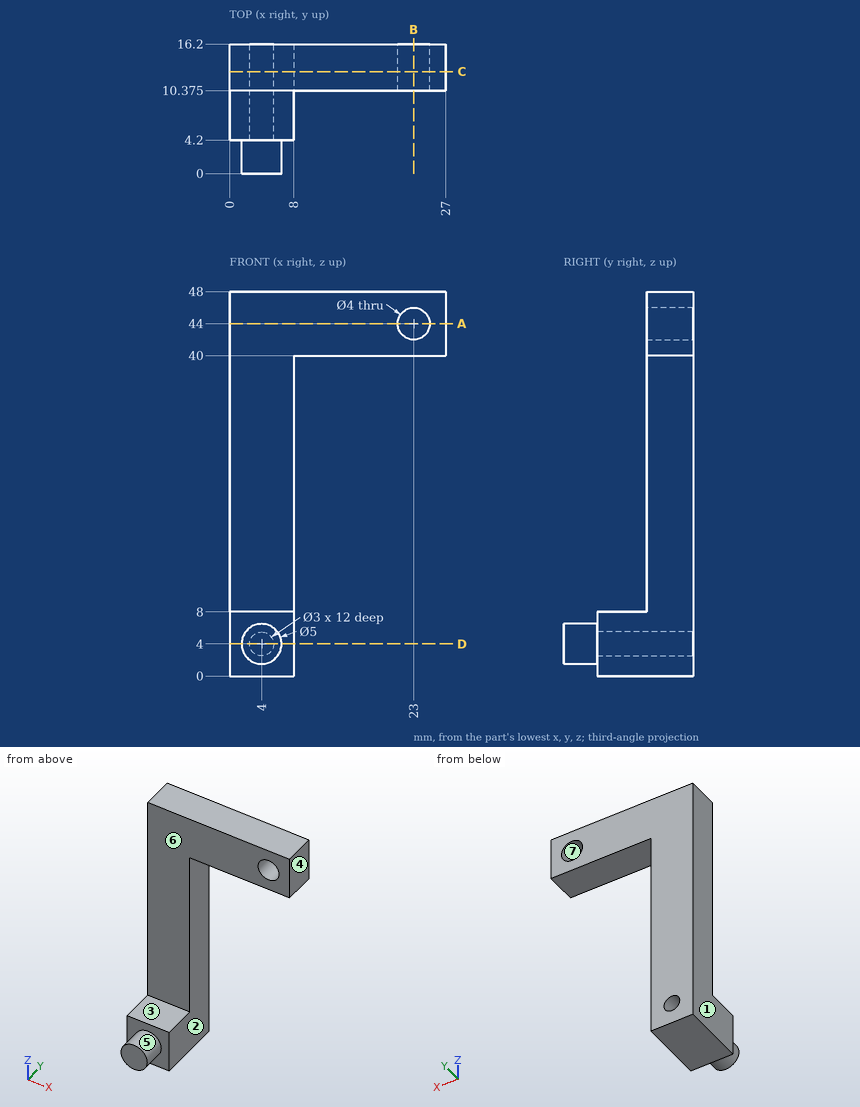
Geometry check sheet. Reference: drawing and pictorial views, mm from the part's lowest x, y, z. A direction names the side the tool comes from. Coordinates: 2 decimals unless noted, no trailing zeros. Order: outer loops, then holes, each group sorted by start corner. A loop starts at its lowest first (then second) coordinate and runs counter-clockwise, first axis right, second up. Notation, with made-up numbers: (-23, -5) -> (0, -5) arc R30 cw to (0, 17) -> close; hole circle Ø2 at (47, 89.25). An arc over 180 degrees is marked (long way). Put each result on its own line as item: value. Start each with the question number.
1) Cross-section at A-A (z = 44). Enter the section's corners in (x, y) (3 decimals), plus the area to 3 significant figures.
2) Cross-section at C-C (y = 12.75). Enter the section's corners in (x, z), plus the area to 3 significant figures.
3) Cross-section at D-D (z = 4). Enter the section's corners in (x, y).
4) Tool access check on the marked faces 1, 2 and 3. Record the directions out of +Z, -Z, +X, -X, +Y, -Y that give a thin tool (end or side, any length) a straight path to the whole face; none if there is none.
5) Material ranges on L1, parallel to X at y = 10.75, z = 4; L2, parallel to X at y = 12.75, z = 44; L3, parallel to Y at x = 16.25, z = 41 (3 decimals), recorded low to high.
6) Go/stop test with flat-tipped pins: pin 1 (3 mm diameter, centred on x = 3.5, y = 7.5, fed in from +Z); pin 2 (3.5 mm diameter, centred on y = 11.5, z = 13.5, fed in from +X); pin 3 (5 mm diameter, centred on x = 9.5, z = 6, fed in from -Y). Record where each tip stops, or that it passes through.
7) Release check for a two-part mould opening along X. For the marked faces 4, 5, 6 and 7 record: pulls with the +X half, pulls with the -X half, needs draft (parallel to the pull), parting line crosses it, or undercut.
8) Cross-section at B-B (x = 23). Enter the section's corners in (y, z) (3 decimals).
Geometry check:
1. outline: (0, 10.375) -> (21, 10.375) -> (21, 16.2) -> (0, 16.2) -> close; (25, 10.375) -> (27, 10.375) -> (27, 16.2) -> (25, 16.2) -> close
1. area: 134 mm^2
2. outline: (0, 0) -> (8, 0) -> (8, 40) -> (27, 40) -> (27, 48) -> (0, 48) -> close; hole circle Ø3 at (4, 4); hole circle Ø4 at (23, 44)
2. area: 516 mm^2
3. outline: (0, 4.2) -> (1.5, 4.2) -> (1.5, 0) -> (6.5, 0) -> (6.5, 4.2) -> (8, 4.2) -> (8, 16.2) -> (5.5, 16.2) -> (5.5, 4.2) -> (2.5, 4.2) -> (2.5, 16.2) -> (0, 16.2) -> close
4. face 1: +Z, -Z, -X, +Y, -Y
4. face 2: -Z, +X, +Y, -Y
4. face 3: +Z, +X, -X, -Y
5. L1: x = 0 to 2.5, 5.5 to 8
5. L2: x = 0 to 21, 25 to 27
5. L3: y = 10.375 to 16.2
6. pin 1: stops at z = 8
6. pin 2: stops at x = 8
6. pin 3: stops at y = 4.2
7. face 4: pulls with the +X half
7. face 5: parting line crosses it
7. face 6: needs draft
7. face 7: undercut
8. outline: (10.375, 40) -> (16.2, 40) -> (16.2, 42) -> (10.375, 42) -> close; (10.375, 46) -> (16.2, 46) -> (16.2, 48) -> (10.375, 48) -> close
